Part model, mm, in its own coordinate system. A direction names the side the tool comes from. Give positions to 0.01 mm unless a question says otherwise; leave off trailing zeros. Write each loop counter-clockwise with the first axis right and the second up, starting at its lowest first coordinate (ties: lowest second). Pieces come first, ordered by that corner, then holes. Notation, with made-up numbers: (-31.75, 43) - (-23.75, 43) arc R17 cw to (-23.75, 67) - close; hole circle Ø10 at (54.5, -14.75). An arc over 180 degrees is marked (long way). Answer in a Markdown table with one row per item. Add a question column.
1. Band-saw the part on C-C on z = -14.5. Write the cut outline in (x, y).
2. Probe line 1 along X through (y, z) = (-0.25, 6.5); line 2 along X through (y, z) = (3.25, 1); line 3 along Z through (x, y) = (-11.5, -1.5). List the from-to ranges inside material, lowest first.
3. Band-saw the part on D-D on z = 18.5. Write the cut outline in (x, y), plus the area to 3 significant figures.
4. Drop flat-ended pins along their axis: pin 1 Ø3 at (x, y) = (3, 1) entering from +Z; pin 2 Ø2.5 at (y, z) = (-1, -17) entering from -X; pin 3 Ø2.5 at (y, z) = (1, -0.5) entering from -X. Give the stop position or say it passes through.
5. Band-saw the part on B-B on x = 0. Write the cut outline in (y, z), plus the area to 3 significant figures.
6. Which spindle directions (+Z, -Z, +X, -X, +Y, -Y) get a long thin tool onto all of the face, cutting with end or side? Do faces 1 (the cylindrical face through (-7.7, 2.8, 0)), 2 (the flat face through (2, 0, -3.8)), 3 (the flat face through (-11.431, -1.676, -7.697)). Say none if no direction does.
```python
from build123d import *

# Parameters (mm, degrees)
ESBO_O1_R                              = 22.95
RESSALTO_EXTRUS_O1_DEPTH               = 3.4
ESBO_O2_R                              = 22.95
RESSALTO_EXTRUS_O2_DEPTH               = 2.266666667
CORTE_EXTRUS_O1_DEPTH                  = 7.8
CHANFRO1_SIZE                          = 1
RESSALTO_EXTRUS_O3_DEPTH               = 6.8
FURO_DE_DI_METRO_5_6_5_6_1_D           = 5.6
FURO_DE_DI_METRO_5_6_5_6_1_DEPTH       = 10
FURO_DE_DI_METRO_5_6_5_6_1_CSINK_D     = 5.65
FURO_DE_DI_METRO_5_6_5_6_1_CSINK_ANGLE = 90
FURO_DE_DI_METRO_5_6_5_6_1_TIP         = 1.682409733
ESBO_O8_W                              = 7.937144563
ESBO_O8_H                              = 2.1
CORTE_EXTRUS_O2_DEPTH                  = 4.2


with BuildPart() as part:
    # Esboço1 → Ressalto-extrusão1 (new body, symmetric)
    with BuildSketch(Plane(origin=(0, 0, 0), x_dir=(1, 0, 0), z_dir=(0, 1, 0))):
        Circle(ESBO_O1_R)
        with BuildLine():
            Line((-7.092448526, 2.997861554), (-17.819307423, 9.191016426))
            ThreePointArc((-17.819307423, 9.191016426), (-20.05, 0), (-17.819307423, -9.191016426))
            Line((-17.819307423, -9.191016426), (-7.092448526, -2.997861554))
            ThreePointArc((-7.092448526, -2.997861554), (-7.7, 0), (-7.092448526, 2.997861554))
        make_face(mode=Mode.SUBTRACT)
        with BuildLine():
            Line((-6.142448526, 4.643309822), (-16.869307423, 10.836464693))
            ThreePointArc((-16.869307423, 10.836464693), (-10.025, 17.363809346), (-0.95, 20.02748112))
            Line((-0.95, 20.02748112), (-0.95, 7.641171376))
            ThreePointArc((-0.95, 7.641171376), (-3.85, 6.668395609), (-6.142448526, 4.643309822))
        make_face(mode=Mode.SUBTRACT)
        with BuildLine():
            Line((0.95, 7.641171376), (0.95, 20.02748112))
            ThreePointArc((0.95, 20.02748112), (10.025, 17.363809346), (16.869307423, 10.836464693))
            Line((16.869307423, 10.836464693), (6.142448526, 4.643309822))
            ThreePointArc((6.142448526, 4.643309822), (3.85, 6.668395609), (0.95, 7.641171376))
        make_face(mode=Mode.SUBTRACT)
        with BuildLine():
            Line((7.092448526, 2.997861554), (17.819307423, 9.191016426))
            ThreePointArc((17.819307423, 9.191016426), (20.05, 0), (17.819307423, -9.191016426))
            Line((17.819307423, -9.191016426), (7.092448526, -2.997861554))
            ThreePointArc((7.092448526, -2.997861554), (7.7, 0), (7.092448526, 2.997861554))
        make_face(mode=Mode.SUBTRACT)
        with BuildLine():
            Line((6.142448526, -4.643309822), (16.869307423, -10.836464693))
            ThreePointArc((16.869307423, -10.836464693), (10.025, -17.363809346), (0.95, -20.02748112))
            Line((0.95, -20.02748112), (0.95, -7.641171376))
            ThreePointArc((0.95, -7.641171376), (3.85, -6.668395609), (6.142448526, -4.643309822))
        make_face(mode=Mode.SUBTRACT)
        with BuildLine():
            Line((-0.95, -7.641171376), (-0.95, -20.02748112))
            ThreePointArc((-0.95, -20.02748112), (-10.025, -17.363809346), (-16.869307423, -10.836464693))
            Line((-16.869307423, -10.836464693), (-6.142448526, -4.643309822))
            ThreePointArc((-6.142448526, -4.643309822), (-3.85, -6.668395609), (-0.95, -7.641171376))
        make_face(mode=Mode.SUBTRACT)
    extrude(amount=RESSALTO_EXTRUS_O1_DEPTH, both=True)

    # Esboço2 → Ressalto-extrusão2 (add)
    with BuildSketch(Plane(origin=(0, 0, 0), x_dir=(1, 0, 0), z_dir=(0, 1, 0))):
        Circle(ESBO_O2_R)
    extrude(amount=RESSALTO_EXTRUS_O2_DEPTH)

    # Esboço3 → Corte-extrusão1 (cut, through all)
    with BuildSketch(Plane(origin=(0, 3.4, 0), x_dir=(1, 0, 0), z_dir=(0, 1, 0))):
        with BuildLine():
            Line((1.00475453, 3.8), (3.85, 3.8))
            Line((3.85, 3.8), (3.85, -3.8))
            Line((3.85, -3.8), (-3.85, -3.8))
            Line((-3.85, -3.8), (-3.85, 3.8))
            Line((-3.85, 3.8), (-1.00475453, 3.8))
            ThreePointArc((-1.00475453, 3.8), (0, 4.80475453), (1.00475453, 3.8))
        make_face()
    extrude(amount=-CORTE_EXTRUS_O1_DEPTH, mode=Mode.SUBTRACT)

    # Chanfro1
    chanfro1_edges = [part.edges().sort_by_distance(p)[0] for p in [
        (3.85, -3.4, 0),
        (0, -3.4, 3.8),
        (-3.85, -3.4, 0),
        (-2.427377265, -3.4, -3.8),
        (0, -3.4, -4.80475453),
        (2.427377265, -3.4, -3.8),
        (3.85, 3.4, 0),
        (2.427377265, 3.4, -3.8),
        (0, 3.4, -4.80475453),
        (-2.427377265, 3.4, -3.8),
        (-3.85, 3.4, 0),
        (0, 3.4, 3.8),
    ]]
    chamfer(chanfro1_edges, length=CHANFRO1_SIZE)

    # Esboço4 → Ressalto-extrusão3 (add)
    with BuildSketch(Plane(origin=(0, 3.4, 0), x_dir=(1, 0, 0), z_dir=(0, 1, 0))):
        with BuildLine():
            Line((9.207366783, 17.810864576), (11.916766484, 23.05196687))
            ThreePointArc((11.916766484, 23.05196687), (24.902926978, 7.297035556), (22.473359228, -12.975))
            ThreePointArc((22.473359228, -12.975), (13.660702639, -12.504832962), (19.233912303, -5.66207714))
            ThreePointArc((19.233912303, -5.66207714), (18.438311669, 7.875986466), (9.207366783, 17.810864576))
        make_face()
    extrude(amount=-RESSALTO_EXTRUS_O3_DEPTH)

    # Furo de diâmetro Ø5.6 (5.6)1
    with Locations(Plane(origin=(0, 3.4, 0), x_dir=(1, 0, 0), z_dir=(0, 1, 0))):
        with Locations((18.186533479, -10.5)):
            CounterSinkHole(FURO_DE_DI_METRO_5_6_5_6_1_D / 2, FURO_DE_DI_METRO_5_6_5_6_1_CSINK_D / 2, depth=FURO_DE_DI_METRO_5_6_5_6_1_DEPTH, counter_sink_angle=FURO_DE_DI_METRO_5_6_5_6_1_CSINK_ANGLE)
            with Locations((0, 0, -(FURO_DE_DI_METRO_5_6_5_6_1_DEPTH + FURO_DE_DI_METRO_5_6_5_6_1_TIP / 2))):  # 118° drill point
                Cone(0, FURO_DE_DI_METRO_5_6_5_6_1_D / 2, FURO_DE_DI_METRO_5_6_5_6_1_TIP, mode=Mode.SUBTRACT)

    # Varredura de corte1: sweep along a path in Esboço7
    with BuildLine(Plane(origin=(0, 0, 0), x_dir=(1, 0, 0), z_dir=(0, 1, 0))) as varredura_de_corte1_path:
        ThreePointArc((19.875283017, -11.475), (19.875283017, 11.475), (0, 22.95))
    # Esboço8 → Varredura de corte1 (sweep, cut)
    with BuildSketch(Plane(origin=(0, 0, 0), x_dir=(0, 0, -1), z_dir=(1, 0, 0))):
        with Locations((26.918572282, 0.25)):
            Rectangle(ESBO_O8_W, ESBO_O8_H)
    sweep(path=varredura_de_corte1_path.line, mode=Mode.SUBTRACT)

    # Esboço9 → Corte-extrusão2 (cut)
    with BuildSketch(Plane(origin=(0, 3.4, 0), x_dir=(1, 0, 0), z_dir=(0, 1, 0))):
        Polygon((18.147037743, -11.574162637), (23.041410617, -14.399930134), (24.539064474, -13.070669968), (18.226029216, -9.425837363), align=None)
    extrude(amount=-CORTE_EXTRUS_O2_DEPTH, mode=Mode.SUBTRACT)


solid = part.part
```
Values:
| question | item | result |
|---|---|---|
| 1 | outline | (-17.79, -3.4) - (-13.85, -3.4) - (-13.85, 0) - (-0.95, 0) - (-0.95, -3.4) - (0.95, -3.4) - (0.95, 0) - (13.85, 0) - (13.85, -3.4) - (21.52, -3.4) - (21.52, -0.8) - (17.79, -0.8) - (17.79, 1.3) - (21.52, 1.3) - (21.52, 3.4) - (13.85, 3.4) - (13.85, 2.27) - (0.95, 2.27) - (0.95, 3.4) - (-0.95, 3.4) - (-0.95, 2.27) - (-13.85, 2.27) - (-13.85, 3.4) - (-17.79, 3.4) - close |
| 2 | line 1 | x = -22.01 to -18.97, -13.16 to -9.36, -4.13 to 4.13, 9.36 to 13.16, 15.27 to 22.01 |
| 2 | line 2 | x = -22.93 to -20.03, -7.63 to -4.7, 4.7 to 7.63, 20.03 to 25.93 |
| 2 | line 3 | z = -19.86 to -16.42, -7.74 to -5.54, 5.54 to 7.74, 16.42 to 19.86 |
| 3 | outline | (-13.58, -3.4) - (-7.73, -3.4) - (-7.73, 0) - (-0.95, 0) - (-0.95, -3.4) - (0.95, -3.4) - (0.95, 0) - (7.73, 0) - (7.73, -3.4) - (13.58, -3.4) - (13.58, 3.4) - (7.73, 3.4) - (7.73, 2.27) - (0.95, 2.27) - (0.95, 3.4) - (-0.95, 3.4) - (-0.95, 2.27) - (-7.73, 2.27) - (-7.73, 3.4) - (-13.58, 3.4) - close |
| 3 | area | 123 mm² |
| 4 | pin 1 | stops at z = 22.9 |
| 4 | pin 2 | stops at x = -16.69 |
| 4 | pin 3 | stops at x = -22.95 |
| 5 | outline | (-3.4, -22.95) - (3.4, -22.95) - (3.4, -5.8) - (2.4, -4.8) - (-2.4, -4.8) - (-3.4, -5.8) - close; (-3.4, 4.8) - (-2.4, 3.8) - (2.4, 3.8) - (3.4, 4.8) - (3.4, 22.95) - (-3.4, 22.95) - close |
| 5 | area | 252 mm² |
| 6 | face 1 | +Y |
| 6 | face 2 | +Y, -Y |
| 6 | face 3 | -Y |
